from build123d import *

# Parameters (mm, degrees)
SKETCH2_R           = 5
SKETCH2_W           = 6.8
SKETCH2_H           = 4
SKETCH2_W_2         = 4
SKETCH2_H_2         = 6.8
BOSS_EXTRUDE1_DEPTH = 10
SKETCH2_4_R         = 5
BOSS_EXTRUDE3_DEPTH = 50
BOSS_EXTRUDE4_START = -40
SKETCH2_5_R         = 5
BOSS_EXTRUDE4_DEPTH = 40


with BuildPart() as part:
    # Sketch2 → Boss-Extrude1 (new body)
    with BuildSketch(Plane.XY):
        Circle(SKETCH2_R)
        with Locations((-3.4, 0)):
            Rectangle(SKETCH2_W, SKETCH2_H)
        with Locations((0, 3.4)):
            Rectangle(SKETCH2_W_2, SKETCH2_H_2)
    extrude(amount=BOSS_EXTRUDE1_DEPTH)

    # Sketch2_4 → Boss-Extrude3 (add)
    with BuildSketch(Plane.XY):
        with Locations(Location((0, 0, 0), (0, 0, 156.421821522))):
            Circle(SKETCH2_4_R)
    extrude(amount=BOSS_EXTRUDE3_DEPTH)

    # Sketch2_5 → Boss-Extrude4 (add)
    with BuildSketch(Plane.XY.offset(BOSS_EXTRUDE4_START)):
        Circle(SKETCH2_5_R)
    extrude(amount=BOSS_EXTRUDE4_DEPTH)


solid = part.part
The listing builds one solid part. Answer for the finished solid, in the listing's coordinates (mm). A direction names the side the tool comes from. Round coordinates to 2 decimals unless told otherwise and drop trailing zeros. Write each loop counter-clockwise with the first axis right and the second up, starting at its lowest first coordinate (ties: lowest second). Pieces come first, ordered by that corner, then holes. Notation, with made-up numbers: (76, 62) - (134, 62) arc R33 ccw to (134, 97) - close; hole circle Ø7 at (-10, -15). An arc over 180 degrees is marked (long way). Use one line per item in the form item = value. Start each with the question number.
Item 1: Find the intervals of material crossed by line 1 (X direction, y = -0.25, z = 11); line 2 (Z direction, x = -5.25, y = 1); line 3 (X direction, y = 2, z = -4.5), in increasing order. Write a range as [from, to].
Item 2: A tool of negligible diameter and unlimited length cuts with its end or side. For faces 4 (the flat face through (2, 6, 5)), 5 (the cylindrical face through (-0.685, -4.953, 4.37)), 6 (the flat face through (0, 0, 50)), 7 (the flat face through (-6, -2, 5)), 8 (the flat face through (-2, 6, 5)), from which of +Z, -Z, +X, -X, +Y, -Y can it reach the whole face along a straight path? Write none if from no direction.
Item 3: Determine the mould class of faces 1 (the flat face through (-6, 2, 5)), 2 (the flat face through (0, 6, 10)), 3 (the flat face through (0, 6, 0)) for opening direction Z: +Z half, -Z half, draft (parallel to the pull), parting line (faces both ways), or undercut.
Item 4: A cutting plane is placed at B-B (z = 30.5). Write down the section's boundary in (x, y).
Item 5: A cutting plane is placed at A-A (z = 4.5). Write down the section's boundary in (x, y).
Item 6: Flat-ended cylindrical pins translate along their axes: pin 1 Ø0.7 at (x, y) = (0.5, 5.5) entering from +Z; pin 2 Ø0.7 at (y, z) = (6, 5) entering from -X; pin 3 Ø6 at (y, z) = (-3.5, 14.5) entering from +X. Find the tip coordinate at first contact, or state that the pin passes through.
The answers:
q1.line_1 = [-4.99, 4.99]
q1.line_2 = [0, 10]
q1.line_3 = [-4.58, 4.58]
q2.face_4 = +Z, -Z, +X, +Y
q2.face_5 = none
q2.face_6 = +Z, +X, -X, +Y, -Y
q2.face_7 = +Z, -Z, -X, -Y
q2.face_8 = +Z, -Z, -X, +Y
q3.face_1 = draft
q3.face_2 = +Z half
q3.face_3 = -Z half
q4.outline = circle Ø10 at (0, 0)
q5.outline = (-6.8, -2) - (-4.58, -2) arc R5 ccw (long way) to (2, 4.58) - (2, 6.8) - (-2, 6.8) - (-2, 4.58) arc R5 ccw to (-4.58, 2) - (-6.8, 2) - close
q6.pin_1 = 10
q6.pin_2 = -2
q6.pin_3 = 4.97
